Check sheet for the drawn part. Datum: minimum x, y, z corner. Units: mm. A direction names the side the tool comes from. Give positions to 0.01 mm unless a question says otherwise; leave off trailing zeros. Order: outer loops, then holes, each group sorted by start corner. A loop starts at its lowest first (then second) coordinate and runs counter-clockwise, first axis right, second up. Notation, with made-up numbers: M -26.75,12 L 18.25,12 A24 ccw 18.25,32 Z; hole C 70,60.25 d2. An arc over 180 degrees is marked long. Put each result on its own line as item: value. Start each with the question number.
Q1. Go/stop test with flat-tipped pins: pin 1 (1.5 mm diameter, centred on y = 14.5, z = 2.5, fed in from -X) (3 decimals); pin 2 (5 mm diameter, centred on x = 13.5, y = 3.5, fed in from -Z). Record where each tip stops, or that it passes through.
Q2. Access from +Z, -Z, +X, -X, +Y, -Y to the whole of each face (thin tool, end or side, straight path). Record for the marked faces 4 and 5.
Q3. Mould release check, pull along Y, two halves, no side actions. Record for the marked faces 1, 2 and 3: +Y half, -Y half, draft (parallel to the pull), parting line (faces both ways), or undercut.
Q4. Section check B-B on y = 10. Record the cut outline in (x, z) (3 decimals), then the cut area to 3 significant figures.
Q5. Section check C-C on z = 18. Record the cut outline in (x, y), then the cut area to 3 significant figures.
Q6. Material ranges on L1, parallel to Y at x = 8, z = 17.65; L2, parallel to X at y = 10, z = 18.75; L3, parallel to X at y = 1, z = 13 (3 decimals), recorded low to high.
Q7. Section check D-D on x = 8. Record the cut outline in (y, z), then the cut area to 3 significant figures.
Q8. Section check A-A on x = 1.5. Record the cut outline in (y, z), then the cut area to 3 significant figures.
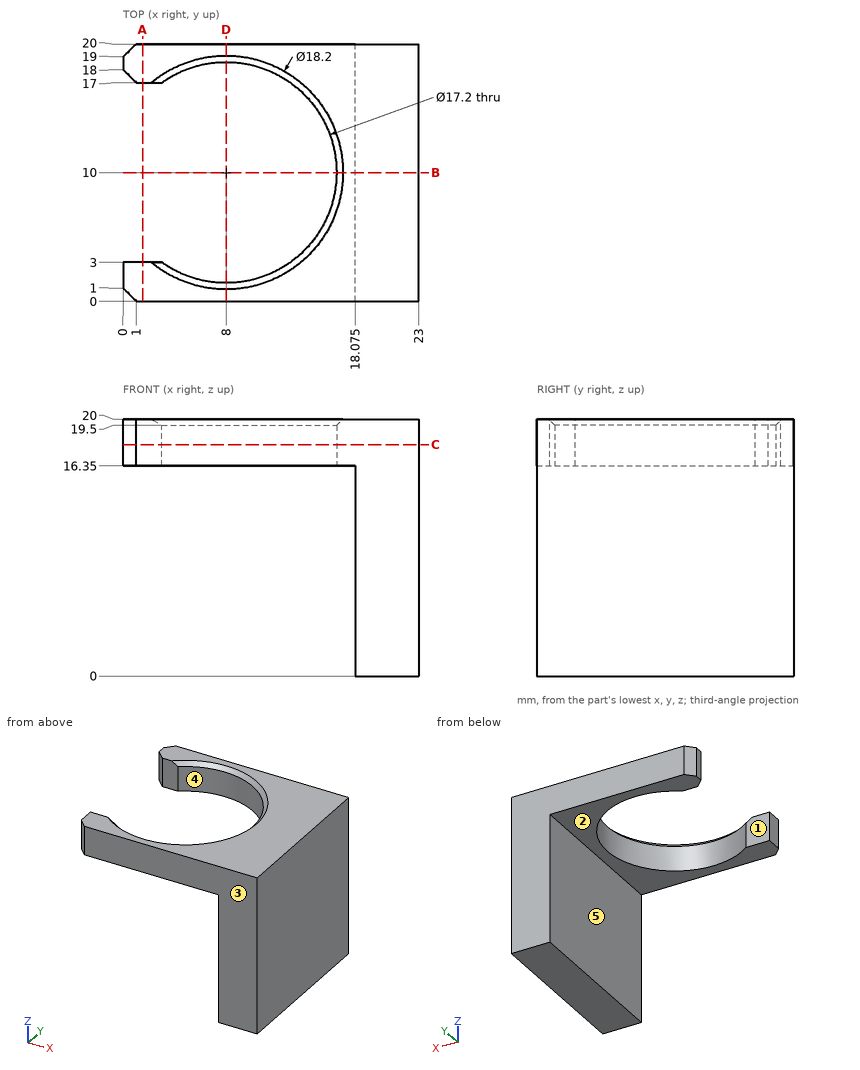
Results found:
1. pin 1: stops at x = 18.075
1. pin 2: stops at z = 16.35
2. face 4: +Z, -Z
2. face 5: -Z, -X, +Y, -Y
3. face 1: undercut
3. face 2: draft
3. face 3: -Y half
4. outline: M 16.6,16.35 L 18.075,16.35 L 18.075,0 L 23,0 L 23,20 L 17.1,20 L 16.6,19.5 Z
4. area: 104 mm^2
5. outline: M 0,1 L 1,0 L 23,0 L 23,20 L 1,20 L 0,19 L 0,18 L 1,17 L 3,17 A8.6 cw long 3,3 L 0,3 Z
5. area: 219 mm^2
6. L1: y = 0 to 1.4, 18.6 to 20
6. L2: x = 16.6 to 23
6. L3: x = 18.075 to 23
7. outline: M 0,16.35 L 1.4,16.35 L 1.4,19.5 L 0.9,20 L 0,20 Z; M 18.6,16.35 L 20,16.35 L 20,20 L 19.1,20 L 18.6,19.5 Z
7. area: 9.97 mm^2
8. outline: M 0,16.35 L 3,16.35 L 3,20 L 0,20 Z; M 17,16.35 L 20,16.35 L 20,20 L 17,20 Z
8. area: 21.9 mm^2
